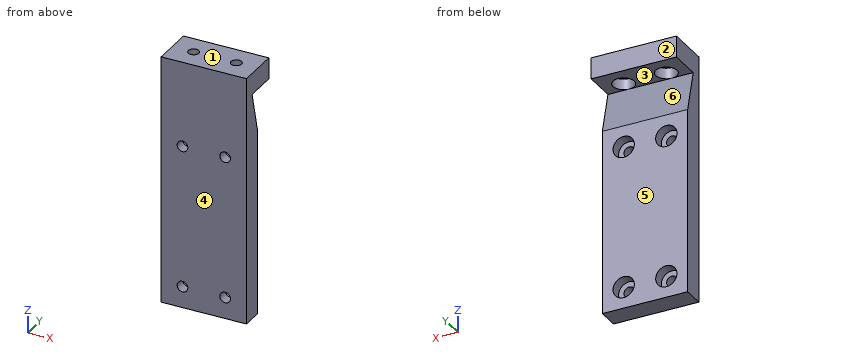
```python
from build123d import *

# Parameters (mm, degrees)
SKETCH1_W               = 40
SKETCH1_H               = 116.7
BOSS_EXTRUDE1_DEPTH     = 10
SKETCH2_W               = 40
SKETCH2_H               = 10
BOSS_EXTRUDE2_DEPTH     = 10
CUT_EXTRUDE1_DEPTH      = 63.487778805
CUT_EXTRUDE1_DEPTH_BACK = 63.487778805
SKETCH3_R               = 2.5
SKETCH4_R               = 5
CUT_EXTRUDE2_DEPTH      = 5
CUT_EXTRUDE3_DEPTH      = 74.516817804
CUT_EXTRUDE3_DEPTH_BACK = 74.516817804
SKETCH6_R               = 2.5
CUT_EXTRUDE4_DEPTH      = 111.385189224
SKETCH7_R               = 5
CUT_EXTRUDE5_DEPTH      = 5


with BuildPart() as part:
    # Sketch1 → Boss-Extrude1 (new body)
    with BuildSketch(Plane(origin=(0, 0, 0), x_dir=(1, 0, 0), z_dir=(0, 1, 0))):
        Rectangle(SKETCH1_W, SKETCH1_H)
    extrude(amount=BOSS_EXTRUDE1_DEPTH)

    # Sketch2 → Boss-Extrude2 (add)
    with BuildSketch(Plane(origin=(0, 10, 0), x_dir=(1, 0, 0), z_dir=(0, 1, 0))):
        with Locations((0, -53.35)):
            Rectangle(SKETCH2_W, SKETCH2_H)
    extrude(amount=BOSS_EXTRUDE2_DEPTH)

    # Sketch3 → Cut-Extrude1 (cut, two sides: drawn at the far end of the back side and taken through both)
    with BuildSketch(Plane(origin=(0, 10, 0), x_dir=(1, 0, 0), z_dir=(0, 1, 0)).offset(-CUT_EXTRUDE1_DEPTH_BACK)):
        with Locations(Location((-10, 48.35, 0), (0, 0, 270))):
            Circle(SKETCH3_R)
        with Locations(Location((10, 48.35, 0), (0, 0, 270))):
            Circle(SKETCH3_R)
        with Locations(Location((10, -18.35, 0), (0, 0, 270))):
            Circle(SKETCH3_R)
        with Locations(Location((-10, -18.35, 0), (0, 0, 270))):
            Circle(SKETCH3_R)
    extrude(amount=CUT_EXTRUDE1_DEPTH + CUT_EXTRUDE1_DEPTH_BACK, mode=Mode.SUBTRACT)

    # Sketch4 → Cut-Extrude2 (cut)
    with BuildSketch(Plane(origin=(0, 10, 0), x_dir=(1, 0, 0), z_dir=(0, 1, 0))):
        with Locations(Location((10, 48.35, 0), (0, 0, 270))):
            Circle(SKETCH4_R)
        with Locations(Location((-10, 48.35, 0), (0, 0, 270))):
            Circle(SKETCH4_R)
        with Locations(Location((10, -18.35, 0), (0, 0, 270))):
            Circle(SKETCH4_R)
        with Locations(Location((-10, -18.35, 0), (0, 0, 270))):
            Circle(SKETCH4_R)
    extrude(amount=-CUT_EXTRUDE2_DEPTH, mode=Mode.SUBTRACT)

    # Sketch5 → Cut-Extrude3 (cut, two sides: drawn at the far end of the back side and taken through both)
    with BuildSketch(Plane.ZY.offset(20).offset(-CUT_EXTRUDE3_DEPTH_BACK)):
        Polygon((28.35, 10), (48.35, 5), (48.35, 10), align=None)
    extrude(amount=CUT_EXTRUDE3_DEPTH + CUT_EXTRUDE3_DEPTH_BACK, mode=Mode.SUBTRACT)

    # Sketch6 → Cut-Extrude4 (cut, through all)
    with BuildSketch(Plane(origin=(0, 0, 48.35), x_dir=(-1, 0, 0), z_dir=(0, 0, -1))):
        with Locations((-10, 10)):
            Circle(SKETCH6_R)
        with Locations((10, 10)):
            Circle(SKETCH6_R)
    extrude(amount=-CUT_EXTRUDE4_DEPTH, mode=Mode.SUBTRACT)

    # Sketch7 → Cut-Extrude5 (cut)
    with BuildSketch(Plane(origin=(0, 0, 48.35), x_dir=(-1, 0, 0), z_dir=(0, 0, -1))):
        with Locations((-10, 10)):
            Circle(SKETCH7_R)
        with Locations((10, 10)):
            Circle(SKETCH7_R)
    extrude(amount=-CUT_EXTRUDE5_DEPTH, mode=Mode.SUBTRACT)


solid = part.part
```
Here's how the part is built. I have some questions about the finished solid (model axes, mm). Face numbers are marked on the shaded views. A direction names the side the tool comes from. Coordinates: 2 decimals unless noted, no trailing zeros. Loops run counter-clockwise (first coordinate to the right, second up) from the corner with the lowest first, then second, coordinate; pieces in that order, holes last. Notation, with made-up numbers: M 52,-20.75 L 111,-20.75 A11 cw 111,-6.75 Z; hole C 88,45 d2. An arc over 180 degrees is marked long. One line per item, written item: value.
1. Will these pins go through, and if not, where does the flat tip stop? pin 1 Ø8 at (x, z) = (-10, -48.35) entering from +Y; pin 2 Ø11.5 at (x, z) = (-10, 18.35) entering from +Y; pin 3 Ø4.5 at (x, y) = (2, 12.5) entering from -Z; pin 4 Ø1 at (y, z) = (12, -5) entering from +X.
Geometry says:
pin 1: stops at y = 5
pin 2: stops at y = 10
pin 3: stops at z = 48.35
pin 4: passes through
2. Imagine slicing it at C-C (y = 11.25). List the corners of the cut face in (x, z) for me.
Geometry says:
outline: M -20,48.35 L -14.84,48.35 L -14.84,53.35 L -12.17,53.35 L -12.17,58.35 L -20,58.35 Z; M -7.83,53.35 L -5.16,53.35 L -5.16,48.35 L 5.16,48.35 L 5.16,53.35 L 7.83,53.35 L 7.83,58.35 L -7.83,58.35 Z; M 12.17,53.35 L 14.84,53.35 L 14.84,48.35 L 20,48.35 L 20,58.35 L 12.17,58.35 Z
3. Imagine slicing it at A-A (z = -48.35). List the corners of the cut face in (x, y) for me.
Geometry says:
outline: M -20,0 L -12.5,0 L -12.5,5 L -15,5 L -15,10 L -20,10 Z; M -7.5,0 L 7.5,0 L 7.5,5 L 5,5 L 5,10 L -5,10 L -5,5 L -7.5,5 Z; M 12.5,0 L 20,0 L 20,10 L 15,10 L 15,5 L 12.5,5 Z
4. Thinking about a two-plate mould opening in Z: for the marked faces 1, 2 and 3, which applies, +Z half, -Z half, draft (parallel to the pull), parting line (faces both ways), or undercut?
Geometry says:
face 1: +Z half
face 2: draft
face 3: undercut
5. Please list where these lines run through material, in increasing order: probe 1 along Z at (x, y) = (-10, 2.8); probe 2 along X at (y, z) = (6.35, -48.35); probe 3 along X at (y, z) = (2.35, -48.35).
Geometry says:
probe 1: z = -58.35 to -50.85, -45.85 to 15.85, 20.85 to 58.35
probe 2: x = -20 to -15, -5 to 5, 15 to 20
probe 3: x = -20 to -12.5, -7.5 to 7.5, 12.5 to 20
6. On a 3-axis mill with a long thin cutter (end or side, diameter ignored), from which of +Z, -Z, +X, -X, +Y, -Y can I reach the whole of each face in a straight line? I mean the marked faces 4, 5 and 6. Say none if no direction works.
Geometry says:
face 4: +Z, -Z, +X, -X, -Y
face 5: -Z, +X, -X, +Y
face 6: +X, -X, +Y
7. Imagine slicing it at D-D (x = 8.5). State how many separate pieces and enclosed holes the cut face has, and give its area (3 significant figures).
Geometry says:
separate pieces: 4
enclosed holes: 0
area: 1,010 mm2
8. Imagine slicing it at B-B (y = 2.5). List the corners of the cut face in (x, z) for me, and give its area (3 significant figures).
Geometry says:
outline: M -20,-58.35 L 20,-58.35 L 20,58.35 L -20,58.35 Z; hole C -10,-48.35 d5; hole C -10,18.35 d5; hole C 10,-48.35 d5; hole C 10,18.35 d5
area: 4,590 mm2
